```python
from build123d import *

# Parameters (mm, degrees)
SKETCH_W        = 160
SKETCH_H        = 100
PAD_DEPTH       = 10
PAD008_DEPTH    = 20
SKETCH029_R     = 4.15
POCKET017_DEPTH = 10
SKETCH031_W     = 55
SKETCH031_H     = 10
PAD010_DEPTH    = 20
SKETCH032_R     = 3
PAD011_DEPTH    = 2
SKETCH033_R     = 1.85
POCKET018_DEPTH = 12.001
SKETCH034_R     = 3.25
POCKET019_DEPTH = 5
SKETCH035_W     = 15
SKETCH035_H     = 35
POCKET020_DEPTH = 5.3
SKETCH036_R     = 1.3
POCKET021_DEPTH = 4.701


with BuildPart() as part:
    # Sketch → Pad (new body)
    with BuildSketch(Plane.XY):
        with Locations((80, 50)):
            Rectangle(SKETCH_W, SKETCH_H)
    extrude(amount=PAD_DEPTH)

    # Sketch001 (on Face5 of Pad) → Pad008 (join)
    with BuildSketch(Plane(origin=(0, 0, 0), x_dir=(1, 0, 0), z_dir=(0, 0, -1))):
        Polygon((0, -10), (0, 0), (51, -18.562482), (51, -28.562482), align=None)
        Polygon((160, 0), (160, -10), (109, -28.562482), (109, -18.562482), align=None)
    extrude(amount=PAD008_DEPTH)

    # Sketch029 (on Face2 of Pad008) → Pocket017 (cut)
    with BuildSketch(Plane(origin=(0, 0, 0), x_dir=(1, 0, 0), z_dir=(0, 0, -1))):
        with Locations((71, -59.794095)):
            Circle(SKETCH029_R)
        with Locations((89, -59.794095)):
            Circle(SKETCH029_R)
    extrude(amount=-POCKET017_DEPTH, mode=Mode.SUBTRACT)

    # Sketch031 (on Face6 of Pocket017) → Pad010 (join)
    with BuildSketch(Plane(origin=(0, 100, 0), x_dir=(-1, 0, 0), z_dir=(0, 1, 0))):
        with Locations((-80, 5)):
            Rectangle(SKETCH031_W, SKETCH031_H)
    extrude(amount=PAD010_DEPTH)

    # Sketch032 (on Face17 of Pad010) → Pad011 (join)
    with BuildSketch(Plane(origin=(0, 0, 0), x_dir=(1, 0, 0), z_dir=(0, 0, -1))):
        with Locations((80, -71.294095)):
            Circle(SKETCH032_R)
        with Locations((101.25, -106.449251)):
            Circle(SKETCH032_R)
        with Locations((58.75, -106.449251)):
            Circle(SKETCH032_R)
    extrude(amount=PAD011_DEPTH)

    # Sketch033 (on Face26 of Pad011) → Pocket018 (cut, through all)
    with BuildSketch(Plane(origin=(0, 0, -2), x_dir=(1, 0, 0), z_dir=(0, 0, -1))):
        with Locations((58.75, -106.449251)):
            Circle(SKETCH033_R)
        with Locations((101.25, -106.449251)):
            Circle(SKETCH033_R)
        with Locations((80, -71.294095)):
            Circle(SKETCH033_R)
    extrude(amount=-POCKET018_DEPTH, mode=Mode.SUBTRACT)

    # Sketch034 (on Face5 of Pocket018) → Pocket019 (cut)
    with BuildSketch(Plane.XY.offset(10)):
        with Locations((58.75, 106.449251)):
            Circle(SKETCH034_R)
        with Locations((101.25, 106.449251)):
            Circle(SKETCH034_R)
        with Locations((80, 71.294095)):
            Circle(SKETCH034_R)
    extrude(amount=-POCKET019_DEPTH, mode=Mode.SUBTRACT)

    # Sketch035 (on Face4 of Pocket019) → Pocket020 (cut)
    with BuildSketch(Plane(origin=(0, 0, 0), x_dir=(1, 0, 0), z_dir=(0, 0, -1))):
        with Locations((152.5, -40)):
            Rectangle(SKETCH035_W, SKETCH035_H)
        with Locations((7.5, -40)):
            Rectangle(SKETCH035_W, SKETCH035_H)
    extrude(amount=-POCKET020_DEPTH, mode=Mode.SUBTRACT)

    # Sketch036 (on Face15 of Pocket020) → Pocket021 (cut, through all)
    with BuildSketch(Plane(origin=(0, 0, 5.3), x_dir=(1, 0, 0), z_dir=(0, 0, -1))):
        with Locations((152.5, -31.25)):
            Circle(SKETCH036_R)
        with Locations((152.5, -48.75)):
            Circle(SKETCH036_R)
        with Locations((7.5, -31.25)):
            Circle(SKETCH036_R)
        with Locations((7.5, -48.75)):
            Circle(SKETCH036_R)
    extrude(amount=-POCKET021_DEPTH, mode=Mode.SUBTRACT)


solid = part.part
```
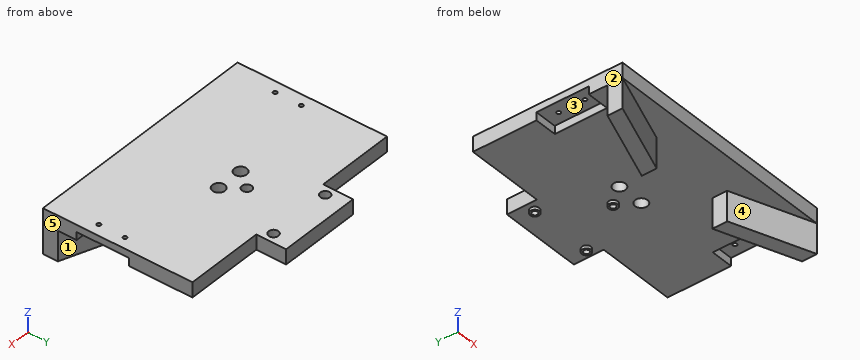
Model file for the job. Use its own axes, mm. Face numbers are marked on the shaded views. A direction names the side the tool comes from. Give positions to 0.01 mm unless a question says otherwise; leave off trailing zeros. Loops run counter-clockwise (first coordinate to the right, second up) from the corner with the lowest first, then second, coordinate; pieces in that order, holes last. Notation, with made-up numbers: (49.25, 34) - (56.25, 34) arc R18 cw to (56.25, 51) - close; hole circle Ø6 at (54.5, 74). An arc over 180 degrees is marked (long way). One line per item, written item: value. Start each with the question number.
1. Probe L1, parallel to X at y = 48.75, z = 8.9; L2, parallel to Y at x = 152.5, z = 6.7; L3, parallel to Y at x = 80, z = 7.2. List the from-to ranges inside material, lowest first. Write a range as from..to.
2. Slice it at D-D (z = 8.25). Give the number of separate pieces and of enclosed holes in the cut face, plus the area to 3 significant figures.
3. Pin check, flat tips, straight feed: pin 1 (2 mm diameter, centred on x = 152.5, y = 48.75, fed in from +Z); pin 2 (2 mm diameter, centred on x = 48, z = -16, fed in from -Y); pin 3 (11 mm diameter, centred on y = 106.5, z = 4, fed in from +X); pin 4 (7.5 mm diameter, centred on x = 152.5, y = 37.5, fed in from -Z). Stop position of each tip, or through.
4. Slice it at A-A (x = 89). List the corners of the cut face in (y, z), plus the area to 3 significant figures.
5. Which spindle directions (+Z, -Z, +X, -X, +Y, -Y) get a long thin tool onto all of the face, cutting with end or side? Do the marked faces 1 and 2. Say none if no direction does.
6. Slice it at C-C (y = 12). List the corners of the cut face in (x, z), plus the area to 3 significant figures.
7. Pull direction X, two halves, no side cores. Call the marked faces 3, 4 and 5: pulls with the +X half, pulls with the -X half, needs draft (parallel to the pull), parting line crosses it, or undercut.
8. Slice it at B-B (z = -6.5). List the corners of the cut face in (x, y), plus the area to 3 significant figures.
Solution:
1. L1: x = 0..6.2, 8.8..151.2, 153.8..160
1. L2: y = 0..29.95, 32.55..47.45, 50.05..100
1. L3: y = 0..68.04, 74.54..120
2. separate pieces: 1
2. enclosed holes: 9
2. area: 16,900 mm^2
3. pin 1: passes through
3. pin 2: stops at y = 17.11
3. pin 3: stops at x = 107.5
3. pin 4: stops at z = 5.3
4. outline: (0, 0) - (55.64, 0) - (55.64, 10) - (0, 10) - close; (63.94, 0) - (120, 0) - (120, 10) - (63.94, 10) - close
4. area: 1,120 mm^2
5. face 1: -Z, +X, +Y
5. face 2: +Z, -Z, -X, +Y, -Y
6. outline: (0, 0) - (5.49, 0) - (5.49, -20) - (32.97, -20) - (32.97, 0) - (127.03, 0) - (127.03, -20) - (154.51, -20) - (154.51, 0) - (160, 0) - (160, 10) - (0, 10) - close
6. area: 2,700 mm^2
7. face 3: needs draft
7. face 4: undercut
7. face 5: pulls with the +X half
8. outline: (0, 0) - (51, 18.56) - (51, 28.56) - (0, 10) - close; (109, 18.56) - (160, 0) - (160, 10) - (109, 28.56) - close
8. area: 1,020 mm^2
